Autodesk Inventor part; units mm, degrees
ref_plane "YZ Plane" through (0, 0, 0) normal (1, 0, 0) x (0, 1, 0)
ref_plane "XZ Plane" through (0, 0, 0) normal (0, 1, 0) x (-1, 0, 0)
ref_plane "XY Plane" through (0, 0, 0) normal (0, 0, 1) x (1, 0, 0)
sketch "Sketch1" plane through (0, 0, 0) normal (0, 0, 1) x (1, 0, 0)
  line L0 (-60, -22.5) -> (60, -22.5)
  line L1 (60, -22.5) -> (60, 22.5)
  line L2 (60, 22.5) -> (-60, 22.5)
  line L3 (-60, 22.5) -> (-60, -22.5)
  line L4 (-60, -22.5) -> (60, 22.5) construction
  line L5 (60, -22.5) -> (-60, 22.5) construction
  circle A0 centre (-25, -7.5) radius 5
  circle A1 centre (25, -7.5) radius 5
  point P0 (0, 0)
  dimension "d0" = 120
  dimension "d1" = 45
  dimension "d2" = 10
  dimension "d3" = 10
  dimension "d4" = 35
  dimension "d5" = 35
  dimension "d6" = 15
  dimension "d7" = 15
extrude "Extrusion1" add sketch "Sketch1" along normal blind 7.9375
chamfer "Chamfer1" distance 7.9375 angle 5 1 edges at (0, 22.5, 7.9375) measured on face at (20, 22.5, 2.6458)
properties part number "Lower blade" material "Steel, Mild"
CAD build for the part. Positions are in the model's coordinates, mm. Give positions to 0.01 mm unless a question says otherwise; leave off trailing zeros. Loops run counter-clockwise (first coordinate to the right, second up) from the corner with the lowest first, then second, coordinate; pieces in that order, holes last. Notation, with made-up numbers: (80, 18) -> (136, 18) arc R15 ccw to (136, 36) -> close; hole circle Ø7 at (-6.75, 6). An arc over 180 degrees is marked (long way). Use a Markdown table: item, result.
1. Wall check: L1, parallel to X at y = -7, z = 6.75; L2, parallel to X at y = -9.5, z = 7.75; L3, parallel to Y at x = 21, z = 7.5. Give the ranges that are in metal, low to high. Write a range as [from, to].
Check result:
| item | result |
|---|---|
| L1 | x = [-60, -29.97], [-20.03, 20.03], [29.97, 60] |
| L2 | x = [-60, -29.58], [-20.42, 20.42], [29.58, 60] |
| L3 | y = [-22.5, -10.5], [-4.5, 21.84] |
2. Slice it at A-A (y = -7.5). List the corners of the cut face in (x, z).
Check result:
| item | result |
|---|---|
| outline | (-60, 0) -> (-30, 0) -> (-30, 7.94) -> (-60, 7.94) -> close; (-20, 0) -> (20, 0) -> (20, 7.94) -> (-20, 7.94) -> close; (30, 0) -> (60, 0) -> (60, 7.94) -> (30, 7.94) -> close |
3. Mould opens along Y. For faces 1 (the flat face through (-1, 0, 0)), 2 (the flat face through (-0.84, 22.15, 4.02)), 3 (the cylindrical face through (-29.995, -7.72, 3.913)) say: pulls with the +Y half, pulls with the -Y half, needs draft (parallel to the pull), parting line crosses it, or undercut.
Check result:
| item | result |
|---|---|
| face 1 | needs draft |
| face 2 | pulls with the +Y half |
| face 3 | undercut |
4. Flat gauge pins, fed straight in: pin 1 (3 mm diameter, centred on x = 4.5, z = 7, fed in from +Y); pin 2 (9 mm diameter, centred on x = -25, y = -7.5, fed in from -Z). Where does each tip first touch, or does it go through?
Check result:
| item | result |
|---|---|
| pin 1 | stops at y = 22.02 |
| pin 2 | passes through |
5. Slice it at C-C (z = 6.5). List the corners of the cut face in (x, y).
Check result:
| item | result |
|---|---|
| outline | (-60, -22.5) -> (60, -22.5) -> (60, 21.93) -> (-60, 21.93) -> close; hole circle Ø10 at (-25, -7.5); hole circle Ø10 at (25, -7.5) |
